Input: part model. Units: mm. Frame: model coordinates. Face numbers are marked on the shaded views. Give positions to 0.01 mm unless a question says otherwise; leave off trailing zeros. Order: outer loops, then holes, each group sorted by start corner. A loop starts at its lowest first (then second) coordinate and runs counter-clockwise, first axis right, second up. Notation, with made-up numbers: M 18,73.25 L 24,73.25 A19 cw 24,84.25 Z; hole C 71.25,75.25 d10. An arc over 180 degrees is marked long. Use a Markdown table: item, result.
from build123d import *

# Parameters (mm, degrees)
SKETCH_1_R      = 1.5
EXTRUDE_1_DEPTH = 3
FILLET_1_R      = 3


with BuildPart() as part:
    # 草图1 → 凸台-拉伸1 (new body)
    with BuildSketch(Plane.XY):
        with BuildLine():
            Line((-7.866463296, 21.612930278), (-4.10424172, 11.276311449))
            ThreePointArc((-4.10424172, 11.276311449), (6.882917236, 9.829824531), (12, 0))
            ThreePointArc((12, 0), (11.817693036, -2.083778132), (11.276311449, -4.10424172))
            Line((11.276311449, -4.10424172), (21.612930278, -7.866463296))
            ThreePointArc((21.612930278, -7.866463296), (22.650578319, -3.993908086), (23, 0))
            ThreePointArc((23, 0), (13.192258036, 18.840497019), (-7.866463296, 21.612930278))
        make_face()
        with Locations((19.25, 0)):
            Circle(SKETCH_1_R, mode=Mode.SUBTRACT)
        with Locations((0, 19.25)):
            Circle(SKETCH_1_R, mode=Mode.SUBTRACT)
    extrude(amount=EXTRUDE_1_DEPTH)

    # 圆角1
    fillet_1_edges = [part.edges().sort_by_distance(p)[0] for p in [
        (11.276311449, -4.10424172, 1.5),
        (-4.10424172, 11.276311449, 1.5),
        (-7.866463296, 21.612930278, 1.5),
        (21.612930278, -7.866463296, 1.5),
    ]]
    fillet(fillet_1_edges, radius=FILLET_1_R)


solid = part.part
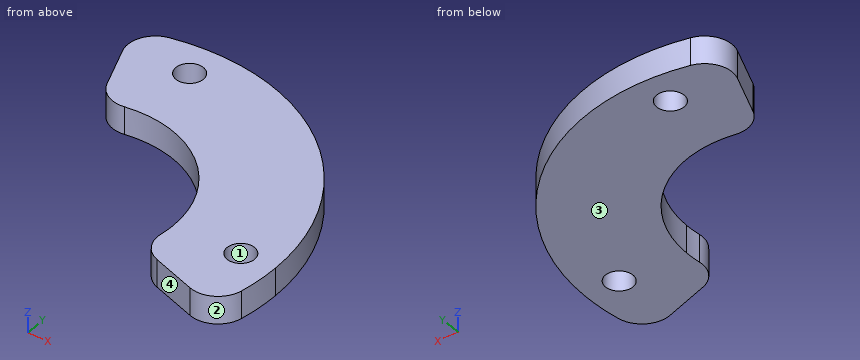
1) Material intervals for line 1 (Y direction, x = 0, z = 2); line 2 (Y direction, x = 19.75, z = 1.8); line 3 (X direction, y = 20.5, z = 1.5), sorted ascending. Write a range as from..to.
Response values:
| item | result |
|---|---|
| line 1 | y = 12..17.75, 20.75..23 |
| line 2 | y = -6.94..-1.41, 1.41..11.79 |
| line 3 | x = -6.81..-0.83, 0.83..10.43 |
2) Cut plane B-B on z = 1.95. Return loops of the section in (x, y).
Response values:
| item | result |
|---|---|
| outline | M -6.76,18.58 L -5.03,13.81 A3 ccw -1.77,11.87 A12 cw 11.87,-1.77 A3 ccw 13.81,-5.03 L 18.58,-6.76 A3 ccw 22.55,-4.54 A23 ccw -4.54,22.55 A3 ccw Z; hole C 0,19.25 d3; hole C 19.25,0 d3 |
3) Cut plane C-C on y = 20. Return loops of the section in (x, z), and give its area (3 significant figures).
Response values:
| item | result |
|---|---|
| outline | M -6.92,0 L -1.3,0 L -1.3,3 L -6.92,3 Z; M 1.3,0 L 11.36,0 L 11.36,3 L 1.3,3 Z |
| area | 47.0 mm² |
4) Mould query, pull axis X, two halves, no side actions, for the marked faces 1, 2, 3 and 4. Classes: released by +X, released by -X, zero draft, split by the parting line, or undercut.
Response values:
| item | result |
|---|---|
| face 1 | undercut |
| face 2 | split by the parting line |
| face 3 | zero draft |
| face 4 | released by -X |
5) Cut plane A-A on x = 0. Return loops of the section in (y, z), and give its area (3 significant figures).
Response values:
| item | result |
|---|---|
| outline | M 12,0 L 17.75,0 L 17.75,3 L 12,3 Z; M 20.75,0 L 23,0 L 23,3 L 20.75,3 Z |
| area | 24.0 mm² |
6) Cut plane D-D on y = 2.5. Return loops of the section in (x, z), and give its area (3 significant figures).
Response values:
| item | result |
|---|---|
| outline | M 11.74,0 L 22.86,0 L 22.86,3 L 11.74,3 Z |
| area | 33.4 mm² |
7) First-contact query: pin 1 Ø10 at (x, y) = (18.5, 14.5) entering from +Z; pin 2 Ø1.5 at (x, z) = (-1, 2.5) entering from +Y. Flat tips, straight axial feed; report the tip coordinate or a pass-through.
Response values:
| item | result |
|---|---|
| pin 1 | stops at z = 3 |
| pin 2 | stops at y = 23 |
